Autodesk Fusion 360 part; units mm, degrees
sketch "Sketch1" plane through (0, 0, 0) normal (0, 1, 0) x (1, 0, 0)
  line L0 (0, -65) -> (0, 55)
  line L1 (-35, 24.9628) -> (-1, 24.9628)
  line L2 (-35, 24.9628) -> (-35, 21.7628)
  arc A0 (-35, 21.7628) -> (-31.4072, 17.5424) centre (-30.7249, 21.7628) ccw
  line L3 (-31.4072, 17.5424) -> (-10, 10)
  line L4 (-10, 10) -> (-7.7084, -4.6955)
  line L5 (0, -5) -> (-3, -5) construction
  line L6 (-7.7084, -4.6955) -> (-3, -5)
  line L7 (-3, -5) -> (-3, 20)
  line L8 (-1, 24.9628) -> (-1, 20)
  line L9 (-1, 20) -> (-3, 20)
  dimension "d1" = 34
  dimension "d2" = 3.2
  dimension "d3" = 3
revolve "Revolve1" add sketch "Sketch1" angle 360 about axis through (0, 0, 65) along (0, 0, -1)
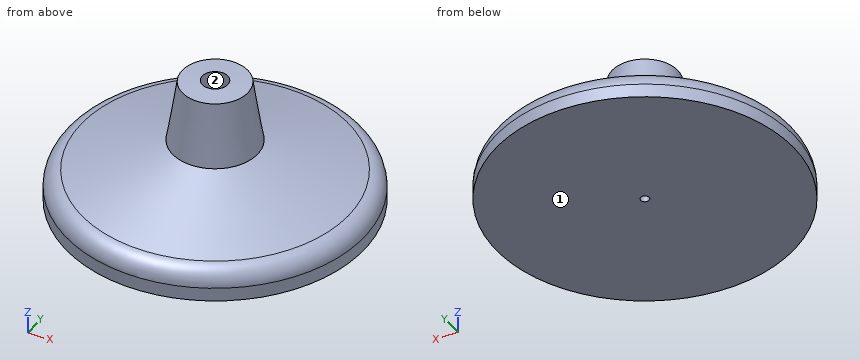
Check sheet for the modelled part. Datum: model origin and axes. Units: mm. Face numbers are marked on the shaded views. A direction names the side the tool comes from. Round coordinates to 2 decimals unless told otherwise and drop trailing zeros. Loops run counter-clockwise (first coordinate to the right, second up) from the corner with the lowest first, then second, coordinate; pieces in that order, holes last. Notation, with made-up numbers: (-14, -34) - (26, -34) arc R14 ccw to (26, -25) - close; hole circle Ø3 at (58, 2.25). An arc over 180 degrees is marked (long way). Write item = value, one per line. Start each with the question number.
Q1. Section check A-A (y = 0). Record the boundary of the cut face in (x, z).
Q2. Thickness scan on L1, parallel to Y at x = 0, z = -21.85; L2, parallel to Z at x = 0.5, y = 2; L3, parallel to Z at x = -18, y = 5. Record the ranges inside material, lowest first.
Q3. Depth check by flat-ended pin: P1, Ø1.5, axis at y = 13, z = -18, coming from the -X side; P2, Ø10, axis at x = -19, y = -22, coming from the +Z side; P3, Ø3, axis at x = -15.5, z = -10, coming from the -Y side; P4, Ø4, axis at y = 23, z = -19.5, coming from the -X side. Enter the tip coordinate at first touch or a pass-through.
Q4. Access from +Z, -Z, +X, -X, +Y, -Y to the whole of each face (thin tool, end or side, straight path). Record for the marked faces 1 and 2.
Q5. Section check C-C (z = -8.75). Record the boundary of the cut face in (x, y), plus the area to 3 significant figures.
Derived:
q1.outline = (-35, -24.96) - (-1, -24.96) - (-1, -20) - (-3, -20) - (-3, 5) - (-7.71, 4.7) - (-10, -10) - (-31.41, -17.54) arc R4.28 ccw to (-35, -21.76) - close; (1, -24.96) - (35, -24.96) - (35, -21.76) arc R4.28 ccw to (31.41, -17.54) - (10, -10) - (7.71, 4.7) - (3, 5) - (3, -20) - (1, -20) - close
q2.L1 = -35 to -1, 1 to 35
q2.L2 = -24.96 to -20
q2.L3 = -24.96 to -13.06
q3.P1 = -31.21
q3.P2 = -14.96
q3.P3 = through
q3.P4 = -27.56
q4.face_1 = -Z, +X, -X, +Y, -Y
q4.face_2 = +Z
q5.outline = circle Ø19.61 at (0, 0); hole circle Ø6 at (0, 0)
q5.area = 274 mm^2
